Design review of the part built by this model. Coordinates are the model's own, in mm. A direction names the side the tool comes from. Give positions to 0.01 mm unless a question says otherwise; leave off trailing zeros. Loops run counter-clockwise (first coordinate to the right, second up) from the corner with the lowest first, then second, coordinate; pieces in that order, holes last. Notation, with made-up numbers: (-12, -9.75) - (17, -9.75) arc R20 cw to (17, 5.25) - close; hole circle Ø9 at (87.5, -36). An arc over 180 degrees is marked (long way). Put each result on its own line as item: value. Start each with the question number.
```python
from build123d import *

# Parameters (mm, degrees)
F1_DEPTH = 45.72
F0_W     = 5.08
F0_H     = 114.3
F2_DEPTH = 6.35
F5_DEPTH = 5.08
F7_DEPTH = 5.08


with BuildPart() as f1:
    # F0 (on Front) → F1 (new body)
    with BuildSketch(Plane.XZ):
        Polygon((-90.17, 29.21), (-95.25, 29.21), (-95.25, 24.13), (-90.17, 24.13), (-2.54, 24.13), (2.54, 24.13), (90.17, 24.13), (95.25, 24.13), (95.25, 29.21), (90.17, 29.21), (2.54, 29.21), (-2.54, 29.21), align=None)
    extrude(amount=F1_DEPTH)


with BuildPart() as f1b:
    # F0 (on Front) → F1, piece 2 (new body)
    with BuildSketch(Plane.XZ):
        Polygon((-90.17, -90.17), (-95.25, -90.17), (-95.25, -95.25), (95.25, -95.25), (95.25, -90.17), (90.17, -90.17), (2.54, -90.17), (-2.54, -90.17), align=None)
    extrude(amount=F1_DEPTH)


with BuildPart() as f2:
    # F0 (on Front) → F2 (new body)
    with BuildSketch(Plane.XZ):
        with Locations((-92.71, -33.02)):
            Rectangle(F0_W, F0_H)
    extrude(amount=F2_DEPTH)


with BuildPart() as f2b:
    # F0 (on Front) → F2, piece 2 (new body)
    with BuildSketch(Plane.XZ):
        Polygon((95.25, 95.25), (-95.25, 95.25), (-95.25, 29.21), (-90.17, 29.21), (-90.17, 90.17), (-2.54, 90.17), (-2.54, 29.21), (2.54, 29.21), (2.54, 90.17), (90.17, 90.17), (90.17, 29.21), (95.25, 29.21), align=None)
    extrude(amount=F2_DEPTH)


with BuildPart() as f2c:
    # F0 (on Front) → F2, piece 3 (new body)
    with BuildSketch(Plane.XZ):
        with Locations((0, -33.02)):
            Rectangle(F0_W, F0_H)
    extrude(amount=F2_DEPTH)


with BuildPart() as f2d:
    # F0 (on Front) → F2, piece 4 (new body)
    with BuildSketch(Plane.XZ):
        with Locations((92.71, -33.02)):
            Rectangle(F0_W, F0_H)
    extrude(amount=F2_DEPTH)


with BuildPart() as f1b_1:
    add(f1b.part)

    # F3: union F1, F2b, F2, F2d, F2c
    add(f1.part)
    add(f2b.part)
    add(f2.part)
    add(f2d.part)
    add(f2c.part)

    # F4 (on face) → F5 (join)
    with BuildSketch(Plane.YZ.offset(95.25)):
        Polygon((-6.35, 61.3136306358), (-45.72, 29.21), (-6.35, 29.21), align=None)
        Polygon((-6.35, -90.17), (-6.35, -58.0663693642), (-45.72, -90.17), align=None)
    extrude(amount=-F5_DEPTH)

    # F6 (on face) → F7 (join)
    with BuildSketch(Plane(origin=(-95.25, 0, 0), x_dir=(0, -1, 0), z_dir=(-1, 0, 0))):
        Polygon((6.35, 29.21), (45.72, 29.21), (6.35, 61.3136306358), align=None)
        Polygon((45.72, -90.17), (6.35, -58.0663693642), (6.35, -90.17), align=None)
    extrude(amount=-F7_DEPTH)


solid = f1b_1.part
```
Item 1: For P1, Ø13.5, axis at x = 30.5, y = -17, coming from the +Z side; P2, Ø23, axis at y = -19.5, z = 56, coming from the +X side; P3, Ø5.5, axis at x = -93, z = -33.5, coming from the -Y side, all flat-tipped, find the tip position at first contact; note any pin that passes through.
Item 2: For L1, parallel to X at y = -5, z = -11; L2, parallel to Z at x = 55.5, y = -37; L3, parallel to X at y = -17, z = 31.5, list the stretches that pass through material, from the lowest coordinate up. Write a range as from..to.
Item 3: Consider section C-C (y = -18). State the section outline as (x, z) points.
Item 4: Machinability: for faces 4 (the flat face through (0, -6.35, -32)), 5 (the flat face through (0, -6.35, 82)), 6 (the flat face through (-2.54, -3, 60)), 7 (the flat face through (93, -6.35, -16)), which of the approach directions +Z, -Z, +X, -X, +Y, -Y give a long, thin tool a straight path to every point of the face, cutting with its end or side? Answer none if there is none.
Item 5: Mouldability with a two-part tool opening along X and no side actions: class faces 1 (the flat face through (1, -23, 29.21)), 2 (the flat face through (-95.25, -6, 0)), 3 (the flat face through (-1, -45.72, 27)) as pulls with the +X half, pulls with the -X half, needs draft (parallel to the pull), parting line crosses it, or undercut.
Item 6: Consider section B-B (x = 65.5). State the section outline as (y, z) points.
Item 7: Consider section A-A (z = 2). State the section outline as (x, y) points.
Item 8: Consider section D-D (y = -30.5). State the section outline as (x, z) points.
Geometry says:
1. P1: stops at z = 29.21
1. P2: stops at x = 95.25
1. P3: stops at y = -6.35
2. L1: x = -95.25..-90.17, -2.54..2.54, 90.17..95.25
2. L2: z = -95.25..-90.17, 24.13..29.21
2. L3: x = -95.25..-90.17, 90.17..95.25
3. outline: (-95.25, -95.25) - (95.25, -95.25) - (95.25, -67.57) - (90.17, -67.57) - (90.17, -90.17) - (-90.17, -90.17) - (-90.17, -67.57) - (-95.25, -67.57) - close; (-95.25, 24.13) - (95.25, 24.13) - (95.25, 51.81) - (90.17, 51.81) - (90.17, 29.21) - (-90.17, 29.21) - (-90.17, 51.81) - (-95.25, 51.81) - close
4. face 4: -Y
4. face 5: +Z, -Y
4. face 6: +Y, -Y
4. face 7: +X, -X, -Y
5. face 1: undercut
5. face 2: pulls with the -X half
5. face 3: needs draft
6. outline: (-45.72, -95.25) - (0, -95.25) - (0, -90.17) - (-45.72, -90.17) - close; (-45.72, 24.13) - (0, 24.13) - (0, 29.21) - (-45.72, 29.21) - close; (-6.35, 90.17) - (0, 90.17) - (0, 95.25) - (-6.35, 95.25) - close
7. outline: (-95.25, -6.35) - (-90.17, -6.35) - (-90.17, 0) - (-95.25, 0) - close; (-2.54, -6.35) - (2.54, -6.35) - (2.54, 0) - (-2.54, 0) - close; (90.17, -6.35) - (95.25, -6.35) - (95.25, 0) - (90.17, 0) - close
8. outline: (-95.25, -95.25) - (95.25, -95.25) - (95.25, -77.76) - (90.17, -77.76) - (90.17, -90.17) - (-90.17, -90.17) - (-90.17, -77.76) - (-95.25, -77.76) - close; (-95.25, 24.13) - (95.25, 24.13) - (95.25, 41.62) - (90.17, 41.62) - (90.17, 29.21) - (-90.17, 29.21) - (-90.17, 41.62) - (-95.25, 41.62) - close
